from build123d import *

# Parameters (mm, degrees)
CUT_EXTRUDE1_DEPTH = 6.35
CIRPATTERN1_COUNT  = 4


with BuildPart() as part:
    # Sketch1 → Revolve1 (revolve)
    with BuildSketch(Plane.XY):
        with BuildLine():
            Line((-7.112, 19.05), (-3.175, 25.4))
            Line((-3.175, 25.4), (-3.175, 57.15))
            Line((-3.175, 57.15), (-7.112, 63.5))
            Line((-7.112, 63.5), (-7.112, 76.2))
            Line((-7.112, 76.2), (-2.413, 76.2))
            Line((-2.413, 76.2), (-2.413, 73.025))
            ThreePointArc((-2.413, 73.025), (0, 70.612), (2.413, 73.025))
            Line((2.413, 73.025), (2.413, 76.2))
            Line((2.413, 76.2), (7.112, 76.2))
            Line((7.112, 76.2), (7.112, 63.5))
            Line((7.112, 63.5), (3.175, 57.15))
            Line((3.175, 57.15), (3.175, 25.4))
            Line((3.175, 25.4), (7.112, 19.05))
            Line((7.112, 19.05), (7.112, 9.55675))
            Line((7.112, 9.55675), (-7.112, 9.55675))
            Line((-7.112, 9.55675), (-7.112, 19.05))
        make_face()
    revolve(axis=Axis((0, 0, 0), (1, 0, 0)))

    # Sketch2 → Cut-Extrude1 (cut)
    with BuildSketch(Plane(origin=(3.175, 0, 0), x_dir=(0, 0, -1), z_dir=(1, 0, 0))):
        with BuildLine():
            Line((23.49644805, 30.621167271), (26.781905408, 34.902858661))
            ThreePointArc((26.781905408, 34.902858661), (27.96426729, 40.046055634), (24.850413368, 44.306849983))
            ThreePointArc((24.850413368, 44.306849983), (0, 50.8), (-24.850413368, 44.306849983))
            ThreePointArc((-24.850413368, 44.306849983), (-27.96426729, 40.046055634), (-26.781905408, 34.902858661))
            Line((-26.781905408, 34.902858661), (-23.49644805, 30.621167271))
            ThreePointArc((-23.49644805, 30.621167271), (-19.797458156, 28.279540119), (-15.462119544, 28.888295471))
            ThreePointArc((-15.462119544, 28.888295471), (0, 32.766), (15.462119544, 28.888295471))
            ThreePointArc((15.462119544, 28.888295471), (19.797458156, 28.279540119), (23.49644805, 30.621167271))
        make_face()
    cut_extrude1 = extrude(amount=-CUT_EXTRUDE1_DEPTH, mode=Mode.SUBTRACT)

    # CirPattern1: Cut-Extrude1 ×4 about axis
    cirpattern1_axis = Axis((0, 0, 0), (1, 0, 0))
    for i in range(1, CIRPATTERN1_COUNT):
        add(cut_extrude1.rotate(cirpattern1_axis, i * 360 / CIRPATTERN1_COUNT), mode=Mode.SUBTRACT)


solid = part.part
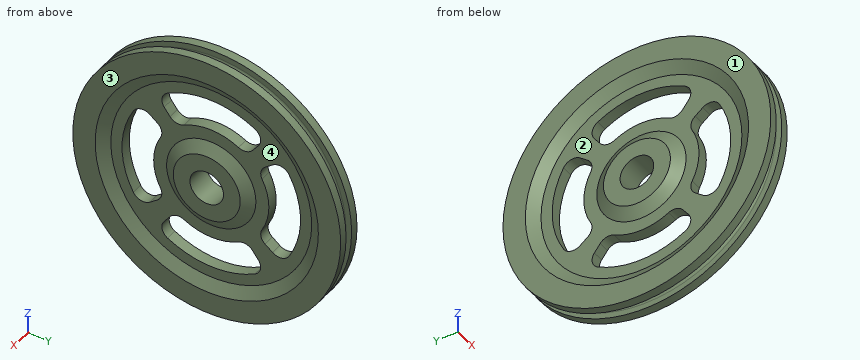
Work out the finished part from the listing and answer in its coordinate system (mm). Face numbers are marked on the shaded views. A direction names the side the tool comes from. Give positions to 0.01 mm unless a question says otherwise; leave off trailing zeros. Order: outer loops, then holes, each group sorted by start corner. A loop starts at its lowest first (then second) coordinate and runs counter-clockwise, first axis right, second up. Notation, with made-up numbers: (3.25, -16.5) - (55.25, -16.5) arc R22 cw to (55.25, 8.5) - close; hole circle Ø7 at (60, -31.5). An arc over 180 degrees is marked (long way). Answer as CSV lines item,"result". Start each with the question number.
Q1. The mould has two halves that part along Z. Classify the marked faces 1 and 2: +Z half, -Z half, draft (parallel to the pull), parting line (faces both ways), or undercut.
Q2. The part is cut by section B-B (x = 5.25). Write down the section's boundary in (y, z).
Q3. For the marked faces 3 and 4, determine the directions among +Z, -Z, +X, -X, +Y, -Y from which every point of the face is accessible in a straight line to the end or side of a thin tool.
Q4. Find the intervals of material crossed by L1, parallel to Z at x = 0.5, y = 0; L2, parallel to Z at x = 0, y = 0; L3, parallel to Z at x = 0.5, y = 15, in increasing order. Write a range as [from, to].
Q5. Given pin 1 Ø11.5 at (y, z) = (0, 0) entering from -X; pin 2 Ø5 at (x, z) = (1.5, 5) entering from -Y; pin 3 Ø8 at (x, z) = (5, -47) entering from -Y; pin 4 Ø1.5 at (x, z) = (0.5, -19) entering from +Y, each flat-ended and moving along its own axis, determine where each tip first touches the part or whether it passes through.
Q6. The part is cut by section A-A (y = 0). Give the number of separate pieces and of enclosed holes in the cut face, then the cut area to 3 significant figures.
Check result:
1,face 1,"draft"
1,face 2,"undercut"
2,outline,"circle Ø152.4 at (0, 0); circle Ø44.11 at (0, 0); hole circle Ø120.99 at (0, 0); hole circle Ø19.11 at (0, 0)"
3,face 3,"+Z, -Z, +X, +Y, -Y"
3,face 4,"+X"
4,L1,"z = [-70.66, -50.8], [-32.77, -9.56], [9.56, 32.77], [50.8, 70.66]"
4,L2,"z = [-70.61, -50.8], [-32.77, -9.56], [9.56, 32.77], [50.8, 70.61]"
4,L3,"z = [-69.05, -48.53], [-29.13, 29.13], [48.53, 69.05]"
5,pin 1,"passes through"
5,pin 2,"stops at y = -76.15"
5,pin 3,"stops at y = -62.91"
5,pin 4,"stops at y = 68.41"
6,separate pieces,"4"
6,enclosed holes,"0"
6,area,"1,020 mm²"
